Here's how the part is built. I have some questions about the finished solid (model axes, mm). Face numbers are marked on the shaded views. A direction names the side the tool comes from. Round coordinates to 2 decimals unless told otherwise and drop trailing zeros. Order: outer loops, then holes, each group sorted by start corner. A loop starts at its lowest first (then second) coordinate and runs counter-clockwise, first axis right, second up. Notation, with made-up numbers: (53, -22.75) -> (65, -22.75) arc R11 cw to (65, -10.75) -> close; hole circle Ø2 at (47.25, 3). An arc over 180 degrees is marked (long way). One line per item, written item: value.
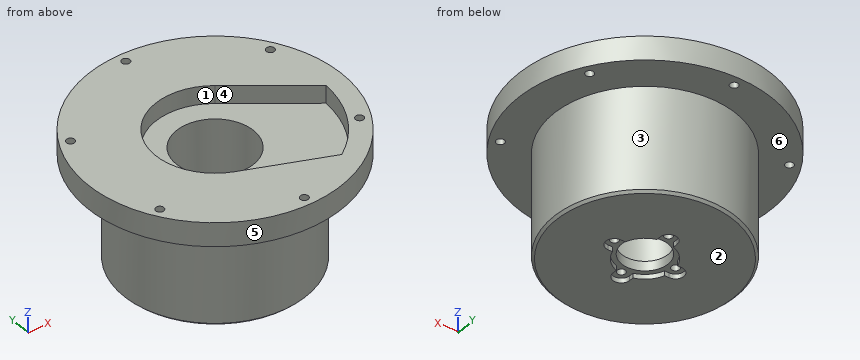
```python
from build123d import *

# Parameters (mm, degrees)
SKETCH1_R            = 53.25
BOSS_EXTRUDE1_DEPTH  = 27
SKETCH2_OUTSIDE_W    = 140.5
SKETCH2_OUTSIDE_H    = 140.5
SKETCH2_OUTSIDE_R    = 38.25
CUT_EXTRUDE1_DEPTH   = 44
M3_CLEARANCE_HOLE2_D = 3.4
CIRPATTERN1_COUNT    = 6
CUT_EXTRUDE3_DEPTH   = 7.5
M3_CLEARANCE_HOLE1_D = 3.4
CUT_EXTRUDE4_DEPTH   = 2
CIRPATTERN2_COUNT    = 4
SKETCH14_R           = 11.7
CUT_EXTRUDE5_DEPTH   = 2
CHAMFER1_SIZE        = 1


with BuildPart() as part:
    # Sketch1 → Boss-Extrude1 (new, symmetric)
    with BuildSketch(Plane.XY):
        Circle(SKETCH1_R)
    extrude(amount=BOSS_EXTRUDE1_DEPTH, both=True)

    # Sketch2 outside → Cut-Extrude1 (cut)
    with BuildSketch(Plane(origin=(0, 0, -27), x_dir=(-1, 0, 0), z_dir=(0, 0, -1))):
        Rectangle(SKETCH2_OUTSIDE_W, SKETCH2_OUTSIDE_H)
        Circle(SKETCH2_OUTSIDE_R, mode=Mode.SUBTRACT)
    extrude(amount=-CUT_EXTRUDE1_DEPTH, mode=Mode.SUBTRACT)

    # M3 Clearance Hole2 (through all)
    with Locations(Plane.XY.offset(27)):
        with Locations((0, 49.125)):
            m3_clearance_hole2 = Hole(M3_CLEARANCE_HOLE2_D / 2)

    # CirPattern1: M3 Clearance Hole2 ×6 about axis
    cirpattern1_axis = Axis((0, 0, 0), (0, 0, 1))
    for i in range(1, CIRPATTERN1_COUNT):
        add(m3_clearance_hole2.rotate(cirpattern1_axis, i * 360 / CIRPATTERN1_COUNT), mode=Mode.SUBTRACT)

    # Sketch6 → Cut-Revolve1 (revolve, cut)
    with BuildSketch(Plane(origin=(0, 0, 0), x_dir=(0, 0, -1), z_dir=(1, 0, 0)), mode=Mode.PRIVATE) as cut_revolve1_sk:
        Polygon((27, 0), (-27, 0), (-27, 16.2), (21, 16.2), (21, 9.7), (27, 9.7), align=None)
    revolve(cut_revolve1_sk.sketch.rotate(Axis((0, 0, -27), (0, 0, 1)), 90), axis=Axis((0, 0, -27), (0, 0, 1)), mode=Mode.SUBTRACT)

    # Sketch11 → Cut-Extrude3 (cut)
    with BuildSketch(Plane.XY.offset(27)):
        with BuildLine():
            Line((-9.567085809, -23.096988313), (25.001320964, -37.415691228))
            ThreePointArc((25.001320964, -37.415691228), (38.97114317, -22.5), (44.903599585, -2.943933469))
            Line((44.903599585, -2.943933469), (15.219035725, 19.833833507))
            ThreePointArc((15.219035725, 19.833833507), (-21.650635095, 12.5), (-9.567085809, -23.096988313))
        make_face()
    extrude(amount=-CUT_EXTRUDE3_DEPTH, mode=Mode.SUBTRACT)

    # M3 Clearance Hole1 (through all)
    with Locations(Plane(origin=(0, 0, -27), x_dir=(-1, 0, 0), z_dir=(0, 0, -1))):
        with Locations((0, 13)):
            m3_clearance_hole1 = Hole(M3_CLEARANCE_HOLE1_D / 2)

    # Sketch13 → Cut-Extrude4 (cut)
    with BuildSketch(Plane(origin=(0, 0, -27), x_dir=(-1, 0, 0), z_dir=(0, 0, -1))):
        with BuildLine():
            Line((-3.55, 13), (-3.55, 9.027042705))
            ThreePointArc((-3.55, 9.027042705), (0, 9.7), (3.55, 9.027042705))
            Line((3.55, 9.027042705), (3.55, 13))
            ThreePointArc((3.55, 13), (0, 16.55), (-3.55, 13))
        make_face()
    cut_extrude4 = extrude(amount=-CUT_EXTRUDE4_DEPTH, mode=Mode.SUBTRACT)

    # CirPattern2: M3 Clearance Hole1, Cut-Extrude4 ×4 about axis
    cirpattern2_axis = Axis((0, 0, 0), (0, 0, 1))
    add([m3_clearance_hole1.rotate(cirpattern2_axis, i * 360 / CIRPATTERN2_COUNT) for i in range(1, CIRPATTERN2_COUNT)], mode=Mode.SUBTRACT)
    add([cut_extrude4.rotate(cirpattern2_axis, i * 360 / CIRPATTERN2_COUNT) for i in range(1, CIRPATTERN2_COUNT)], mode=Mode.SUBTRACT)

    # Sketch14 → Cut-Extrude5 (cut)
    with BuildSketch(Plane(origin=(0, 0, -27), x_dir=(-1, 0, 0), z_dir=(0, 0, -1))):
        Circle(SKETCH14_R)
    extrude(amount=-CUT_EXTRUDE5_DEPTH, mode=Mode.SUBTRACT)

    # Chamfer1
    chamfer1_edges = [part.edges().sort_by_distance(p)[0] for p in [
        (38.25, 0, -27),
    ]]
    chamfer(chamfer1_edges, length=CHAMFER1_SIZE)


solid = part.part
```
Q1. If we mould it in two halves opening along Y, with no side actions, what happens to the marked faces 4, 5 and 6? For each: pulls with the +Y half, pulls with the -Y half, needs draft (parallel to the pull), parting line crosses it, or undercut.
Answers:
face 4: undercut
face 5: parting line crosses it
face 6: needs draft
Q2. I want a section at D-D on y = -45.5. Write out the boundary of the cut face in (x, z), then the cut area to 3 significant figures.
Answers:
outline: (-27.66, 17) -> (27.66, 17) -> (27.66, 27) -> (-27.66, 27) -> close
area: 553 mm2
Q3. Which directions (+Z, -Z, +X, -X, +Y, -Y) give clear straight access to the entire face, cutting with the end or side of a thin tool? Please do the marked faces 1, 2 and 3.
Answers:
face 1: +Z
face 2: -Z, +X, -X, +Y, -Y
face 3: -Z
Q4. I want a section at C-C on x = -46. Write out the boundary of the cut face in (y, z), then the cut area to 3 significant figures.
Answers:
outline: (-26.82, 17) -> (26.82, 17) -> (26.82, 27) -> (-26.82, 27) -> close
area: 536 mm2
Q5. I want a section at B-B on z = 11. Write out the boundary of the cut face in (x, y), then the cut area to 3 significant figures.
Answers:
outline: circle Ø76.5 at (0, 0); hole circle Ø32.4 at (0, 0)
area: 3,770 mm2
Q6. For P1, Ø8, axis at y = -17, z = 8.5, coming from the -X side; P2, Ø3, axis at y = 2.5, z = 8.5, coming from the -X side; P3, Ø1.5, axis at x = 17.5, z = 11.5, coming from the +Y side, each with a flat end and sliding along its axis, tell me the tip position at first contact or that it passes through.
Answers:
P1: x = -35.97
P2: x = -38.24
P3: y = 34.39
Q7. I want a section at A-A on y = 0. Give the number of separate pieces and of enclosed holes in the cut face, then the cut area to 3 significant figures.
Answers:
separate pieces: 4
enclosed holes: 0
area: 2,450 mm2
Q8. I need wall thicknesses on line 1 along Y through (x, z) = (-0.5, 10); line 2 along Y through (x, z) = (-13, -23); line 3 along X through (y, z) = (-14.5, -18). Which ranges of each line are inside material? Lowest first, please.
Answers:
line 1: -38.25 to -16.19, 16.19 to 38.25
line 2: -35.97 to -1.7, 1.7 to 35.97
line 3: -35.4 to -7.22, 7.22 to 35.4
